Verification items for this drawing (mm, ordinates from the low corner). A direction names the side the tool comes from. Round coordinates to 2 decimals unless told otherwise and drop trailing zeros. Loops run counter-clockwise (first coordinate to the right, second up) from the corner with the lowest first, then second, coordinate; pieces in that order, holes last. Notation, with made-up numbers: M 76,20 L 96,20 A17 ccw 96,32 Z; hole C -32,50.25 d6. An arc over 180 degrees is marked long. One line per item, written item: value.
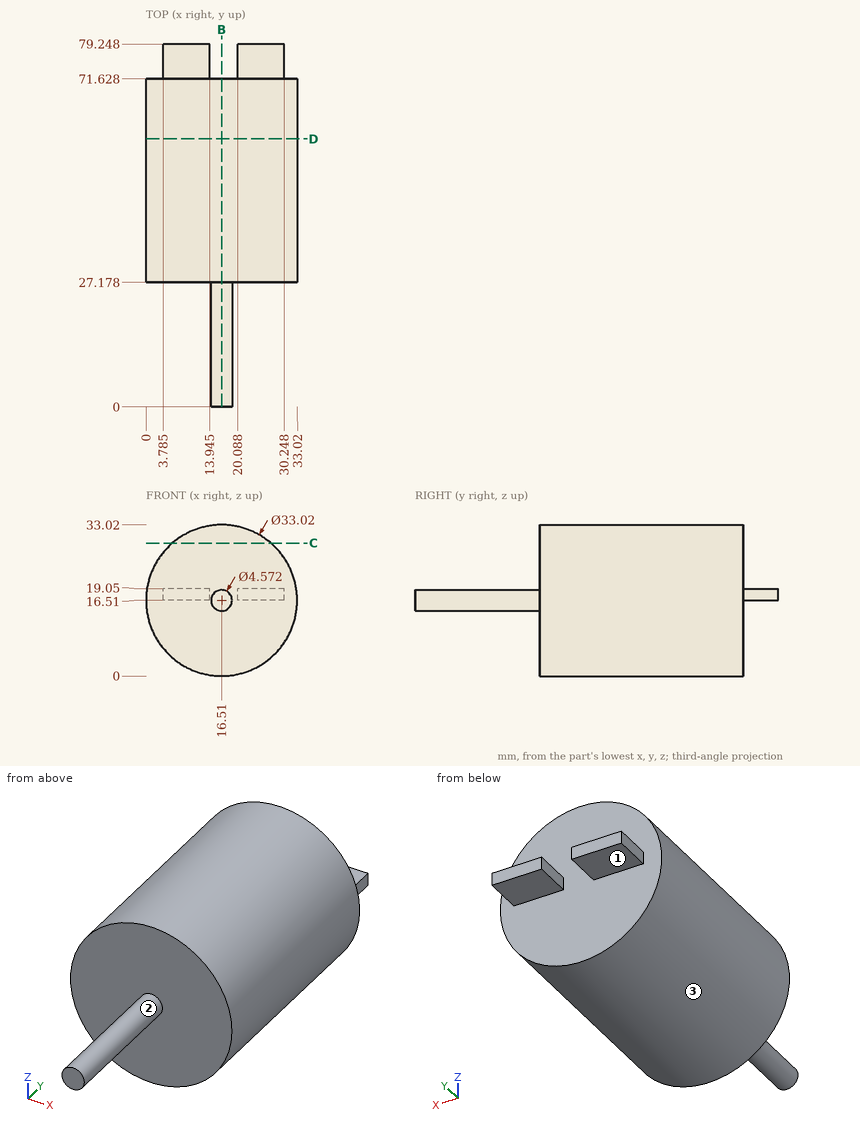
(1) Thickness scan on L1, parallel to Y at x = 4.5, z = 7.5; L2, parallel to Z at x = 16, y = 53.5; L3, parallel to X at y = 50.5, z = 10.5. Record the ranges inside material, lowest first. Write a range as from..to.
Completed:
L1: y = 27.18..71.63
L2: z = 0.01..33.01
L3: x = 1.13..31.89
(2) Sectioned sample at B-B on x = 16.51. Enter the section's corners in (y, z).
Completed:
outline: M 0,14.22 L 27.18,14.22 L 27.18,0 L 71.63,0 L 71.63,33.02 L 27.18,33.02 L 27.18,18.8 L 0,18.8 Z
(3) Sectioned sample at C-C on z = 29. Enter the section's corners in (x, y).
Completed:
outline: M 5.71,27.18 L 27.31,27.18 L 27.31,71.63 L 5.71,71.63 Z
(4) Depth check by flat-ended pin: pin 1 Ø4 at (x, y) = (11.5, 74) entering from +Z; pin 2 Ø4 at (x, y) = (3.5, 54.5) entering from +Z; pin 3 Ø0.8 at (y, z) = (75, 18.5) entering from +X. Enter the tip coordinate at first touch or a pass-through.
Completed:
pin 1: stops at z = 19.05
pin 2: stops at z = 28.81
pin 3: stops at x = 30.25
(5) Tool access check on the marked faces 1, 2 and 3. Record the directions out of +Z, -Z, +X, -X, +Y, -Y that give a thin tool (end or side, any length) a straight path to the whole face; none if there is none.
Completed:
face 1: -Z, +X, -X, +Y
face 2: -Y
face 3: +Y, -Y
(6) Sectioned sample at D-D on y = 58.5. Enter the section's corners in (x, z).
Completed:
outline: C 16.51,16.51 d33.02
